Here's how the part is built. I have some questions about the finished solid (model axes, mm). A direction names the side the tool comes from. Coordinates: 2 decimals unless noted, no trailing zeros. Loops run counter-clockwise (first coordinate to the right, second up) from the corner with the lowest first, then second, coordinate; pieces in that order, holes last.
```python
from build123d import *

# Parameters (mm, degrees)
SKETCH_1_R          = 5
EXTRUDE_1_DEPTH     = 10
SKETCH_2_R          = 10
SKETCH_2_R_2        = 5
EXTRUDE_2_DEPTH     = 16.5
SKETCH_3_R          = 7.75
SKETCH_3_R_2        = 15
CUT_EXTRUDE_1_DEPTH = 15
SKETCH_5_R          = 18.5
CUT_EXTRUDE_3_DEPTH = 10
EXTRUDE_START       = -2
SKETCH_6_R          = 18.5
EXTRUDE_3_DEPTH     = 2
SKETCH_7_R          = 10.1
CUT_EXTRUDE_4_DEPTH = 8


with BuildPart() as part:
    # 草图1 → 凸台-拉伸1 (new body)
    with BuildSketch(Plane.XY):
        with BuildLine():
            ThreePointArc((-128.022678922, -73.913928138), (-90.421378279, 38.440519474), (0, 115))
            ThreePointArc((0, 115), (90.421378279, 38.440519474), (128.022678922, -73.913928138))
            ThreePointArc((128.022678922, -73.913928138), (0, -115), (-128.022678922, -73.913928138))
        make_face()
        with Locations((0, 103)):
            Circle(SKETCH_1_R, mode=Mode.SUBTRACT)
        with Locations((-117.630374076, -67.913928138)):
            Circle(SKETCH_1_R, mode=Mode.SUBTRACT)
        with Locations((117.630374076, -67.913928138)):
            Circle(SKETCH_1_R, mode=Mode.SUBTRACT)
    extrude(amount=EXTRUDE_1_DEPTH)

    # 草图2 → 凸台-拉伸2 (add)
    # profile 1 of 3: a face of its own
    with BuildSketch(Plane.XY.offset(10)):
        with Locations((0, 103)):
            Circle(SKETCH_2_R)
        with Locations((0, 103)):
            Circle(SKETCH_2_R_2, mode=Mode.SUBTRACT)
    # profile 2 of 3: a face of its own
    with BuildSketch(Plane.XY.offset(10)):
        with Locations(Location((-117.630374076, -67.913928138, 0), (0, 0, 179.375778052))):
            Circle(SKETCH_2_R)
        with Locations((-117.630374076, -67.913928138)):
            Circle(SKETCH_2_R_2, mode=Mode.SUBTRACT)
    # profile 3 of 3: a face of its own
    with BuildSketch(Plane.XY.offset(10)):
        with Locations(Location((117.630374076, -67.913928138, 0), (0, 0, 8.696571879))):
            Circle(SKETCH_2_R)
        with Locations((117.630374076, -67.913928138)):
            Circle(SKETCH_2_R_2, mode=Mode.SUBTRACT)
    extrude(amount=EXTRUDE_2_DEPTH)

    # 草图3 → 切除-拉伸1 (cut)
    with BuildSketch(Plane(origin=(0, 0, 0), x_dir=(-1, 0, 0), z_dir=(0, 0, -1))):
        with Locations((-12.650995066, 69.515536741)):
            Circle(SKETCH_3_R)
        with Locations((-82.334125615, -39.530718783)):
            Circle(SKETCH_3_R)
        with Locations((12.428876199, -23.298802993)):
            Circle(SKETCH_3_R_2)
    extrude(amount=-CUT_EXTRUDE_1_DEPTH, mode=Mode.SUBTRACT)

    # 草图5 → 切除-拉伸3 (cut)
    with BuildSketch(Plane(origin=(0, 0, 0), x_dir=(-1, 0, 0), z_dir=(0, 0, -1))):
        with Locations((12.428876199, -23.298802993)):
            Circle(SKETCH_5_R)
    extrude(amount=-CUT_EXTRUDE_3_DEPTH, mode=Mode.SUBTRACT)

    # 草图6 → 凸台-拉伸3 (add)
    with BuildSketch(Plane.XY.offset(10).offset(EXTRUDE_START)):
        with Locations(Location((-12.428876199, -23.298802993, 0), (0, 0, 180))):
            Circle(SKETCH_6_R)
    extrude(amount=EXTRUDE_3_DEPTH)

    # 草图7 → 切除-拉伸4 (cut)
    with BuildSketch(Plane(origin=(0, 0, 8), x_dir=(-1, 0, 0), z_dir=(0, 0, -1))):
        with Locations((12.428876199, -23.298802993)):
            Circle(SKETCH_7_R)
    extrude(amount=-CUT_EXTRUDE_4_DEPTH, mode=Mode.SUBTRACT)


solid = part.part
```
1. For pin 1 (11.5 mm diameter, centred on x = -117.63, y = -67.91, fed in from +Z); pin 2 (4 mm diameter, centred on y = -57.5, z = 19, fed in from -X); pin 3 (4 mm diameter, centred on y = 63, z = 9, fed in from +X); pin 4 (11 mm diameter, centred on x = -7, y = -22.5, fed in from -Z), each with a flat end and sliding along its axis, tell me the tip position at first contact or that it passes through.
2. I want a section at B-B (x = -18). Please give me the cut outline in (y, z), then the cut area to 3 significant figures.
3. We'd pull the mould along X, two halves only. Please class faces 4 (the cylindrical face through (89.47, 39.83, 4.93)), 5 (the cylindrical face through (-110.33, -74.75, 18.13)), 6 (the cylindrical face through (-1.302, 112.915, 18.134)), 7 (the cylindrical face through (113.663, -70.956, 13.064)): +X half, -X half, draft (parallel to the pull), parting line (faces both ways), or undercut.
4. I want a section at C-C (y = 103). Please give me the cut outline in (x, z), then the cut area to 3 significant figures.
5. I need wall thicknesses on line 1 along X through (y, z) = (-64.5, 15.75); line 2 along Y through (x, z) = (0, 13.75); line 3 along Z through (x, y) = (36, 13). Which ranges of each line are inside material? Lowest first, please.
6. I want a section at D-D (z = 3.5). Please give me the cut outline in (x, y), then the cut area to 3 significant figures.
7. I want a section at A-A (z = 19.25). Please give me the cut outline in (x, y), then the cut area to 3 significant figures.
8. On a 3-axis mill with a long thin cutter (end or side, diameter ignored), from which of +Z, -Z, +X, -X, +Y, -Y can I reach the whole of each face in a straight line? I mean faces 1 (the cylindrical face through (126.605, -63.503, 18.134)), 2 (the flat face through (-20, -15, 8)), 3 (the flat face through (2, 108, 26.5)). Say none if no direction works.
Response values:
1. pin 1: stops at z = 26.5
1. pin 2: stops at x = -123.03
1. pin 3: stops at x = 72.89
1. pin 4: stops at z = 8
2. outline: (-114.26, 0) - (-40.94, 0) - (-40.94, 8) - (-31.72, 8) - (-31.72, 10) - (-114.26, 10) - close; (-14.87, 8) - (-5.66, 8) - (-5.66, 0) - (105.72, 0) - (105.72, 10) - (-14.87, 10) - close
2. area: 1,880 mm2
3. face 4: +X half
3. face 5: undercut
3. face 6: parting line
3. face 7: undercut
4. outline: (-22.6, 0) - (-5, 0) - (-5, 26.5) - (-10, 26.5) - (-10, 10) - (-22.6, 10) - close; (5, 0) - (22.6, 0) - (22.6, 10) - (10, 10) - (10, 26.5) - (5, 26.5) - close
4. area: 517 mm2
5. line 1: x = -127.03 to -121.28, -113.98 to -108.23, 108.23 to 113.98, 121.28 to 127.03
5. line 2: y = 93 to 98, 108 to 113
5. line 3: z = 0 to 10
6. outline: (-128.02, -73.91) arc R220 ccw to (128.02, -73.91) arc R220 ccw to (0, 115) arc R220 ccw to start; hole circle Ø10 at (-117.63, -67.91); hole circle Ø37 at (-12.43, -23.3); hole circle Ø10 at (0, 103); hole circle Ø15.5 at (12.65, 69.52); hole circle Ø15.5 at (82.33, -39.53); hole circle Ø10 at (117.63, -67.91)
6. area: 39,500 mm2
7. outline: circle Ø20 at (-117.63, -67.91); circle Ø20 at (0, 103); circle Ø20 at (117.63, -67.91); hole circle Ø10 at (-117.63, -67.91); hole circle Ø10 at (0, 103); hole circle Ø10 at (117.63, -67.91)
7. area: 707 mm2
8. face 1: +Z
8. face 2: -Z
8. face 3: +Z, +X, -X, +Y, -Y
